Source: CAD feature listing. Evaluate the final solid. Frame: model axes, mm. A direction names the side the tool comes from. Give positions to 0.01 mm unless a question says otherwise; leave off trailing zeros. Loops run counter-clockwise (first coordinate to the right, second up) from the corner with the lowest first, then second, coordinate; pieces in that order, holes last. Notation, with made-up numbers: (-35.75, 21.25) -> (-12.75, 21.25) arc R11 cw to (-12.75, 38.25) -> close; hole circle Ø10 at (-12.5, 73.25). An arc over 180 degrees is marked (long way). Put each result on its own line as item: value.
```python
from build123d import *

# Parameters (mm, degrees)
CROQUIS1_R              = 11
CROQUIS1_R_2            = 4
SALIENTE_EXTRUIR1_DEPTH = 3.5
CROQUIS2_R              = 9.5
CROQUIS2_R_2            = 5.5
CORTAR_EXTRUIR1_DEPTH   = 1
CHAFL_N1_SIZE           = 0.3


with BuildPart() as part:
    # Croquis1 → Saliente-Extruir1 (new, symmetric)
    with BuildSketch(Plane.XY):
        Circle(CROQUIS1_R)
        Circle(CROQUIS1_R_2, mode=Mode.SUBTRACT)
    extrude(amount=SALIENTE_EXTRUIR1_DEPTH, both=True)

    # Croquis2 → Cortar-Extruir1 (cut)
    with BuildSketch(Plane.XY.offset(3.5)):
        Circle(CROQUIS2_R)
        Circle(CROQUIS2_R_2, mode=Mode.SUBTRACT)
    cortar_extruir1 = extrude(amount=-CORTAR_EXTRUIR1_DEPTH, mode=Mode.SUBTRACT)

    # Simetría1: Cortar-Extruir1 across plane
    add(cortar_extruir1.mirror(Plane.XY), mode=Mode.SUBTRACT)

    # Chaflán1
    chafl_n1_edges = [part.edges().sort_by_distance(p)[0] for p in [
        (-9.5, 0, 3.5),
        (-5.5, 0, 3.5),
        (-5.5, 0, -3.5),
        (-9.5, 0, -3.5),
    ]]
    chamfer(chafl_n1_edges, length=CHAFL_N1_SIZE)


solid = part.part
```
(1) First-contact query: P1, Ø2, axis at x = -6.5, y = 6.5, coming from the -Z side; P2, Ø1.5, axis at y = -3.5, z = -2.5, coming from the -X side; P3, Ø1, axis at y = -3, z = -1, coming from the -X side; P4, Ø6.5, axis at x = 0, y = 0, coming from the +Z side. Flat tips, straight axial feed; report the tip coordinate or a pass-through.
Calculated:
P1: stops at z = -3.5
P2: stops at x = -10.65
P3: stops at x = -10.71
P4: passes through
(2) Section C-C on z = 1.25. Return loops of the section in (x, y), then the cut area to 3 significant figures.
Calculated:
outline: circle Ø22 at (0, 0); hole circle Ø8 at (0, 0)
area: 330 mm²
(3) Line query: probe 1 along Y at (x, z) = (0, 2.8); probe 2 along Y at (x, z) = (0, -1); probe 3 along Z at (x, y) = (5, -6). Output: solid intervals per line, ascending. Write a range as from..to.
Calculated:
probe 1: y = -11..-9.5, -5.5..-4, 4..5.5, 9.5..11
probe 2: y = -11..-4, 4..11
probe 3: z = -2.5..2.5
(4) Reachability of faces 1 (the flat face through (4, -4, -2.5)), 2 (the cylindrical face through (-0.867, -3.905, -0.049)), 3 (the cylindrical face through (-1.19, -5.37, 2.85)) from +Z, -Z, +X, -X, +Y, -Y: full face, straight path, thin tool, end or side. Return the list, or none.
Calculated:
face 1: -Z
face 2: +Z, -Z
face 3: +Z
(5) Draft query along X for faces 4 (the flat face through (-10, -1, 3.5)), 5 (the cylindrical face through (4.38, -8.43, -2.85)), 6 (the cylindrical face through (-2.38, -10.74, 0.05)). Return one class per face: released by +X, released by -X, zero draft, split by the parting line, or undercut.
Calculated:
face 4: zero draft
face 5: undercut
face 6: split by the parting line
